```python
from build123d import *

# Parameters (mm, degrees)
F1_DEPTH = 101.6
F3_R     = 1.984375
F4_DEPTH = 25.4
F6_R     = 1.984375
F7_DEPTH = 31.75
F8_DEPTH = 25.4
F9_DEPTH = 12.7


with BuildPart() as f1:
    # F0 (on Front) → F1 (new body)
    with BuildSketch(Plane.XZ):
        with BuildLine():
            Line((114.3, 0), (127, 0))
            ThreePointArc((127, 0), (0, 127), (-127, 0))
            Line((-127, 0), (-114.3, 0))
            ThreePointArc((-114.3, 0), (0, 114.3), (114.3, 0))
        make_face()
    extrude(amount=F1_DEPTH)

    # F3 (on face) → F4 (cut)
    with BuildSketch(Plane(origin=(0, 0, 0), x_dir=(1, 0, 0), z_dir=(0, 0, -1))):
        with Locations((0, 222.573593)):
            Circle(F3_R)
    extrude(amount=-F4_DEPTH, mode=Mode.SUBTRACT)

    # F6 (on offset) → F7 (cut)
    with BuildSketch(Plane.YZ.offset(152.4)):
        with Locations((-12.7, 6.35)):
            Circle(F6_R)
    extrude(amount=-F7_DEPTH, mode=Mode.SUBTRACT)

    # F2 (on face) → F8 (join)
    with BuildSketch(Plane(origin=(0, 0, 0), x_dir=(1, 0, 0), z_dir=(0, 0, -1))):
        with BuildLine():
            ThreePointArc((-114.3, 101.6), (0, 215.9), (114.3, 101.6))
            Line((114.3, 101.6), (127, 101.6))
            ThreePointArc((127, 101.6), (0, 228.6), (-127, 101.6))
            Line((-127, 101.6), (-114.3, 101.6))
        make_face()
    extrude(amount=-F8_DEPTH)

    # F3 (on face) → F9 (cut)
    with BuildSketch(Plane(origin=(0, 0, 0), x_dir=(1, 0, 0), z_dir=(0, 0, -1))):
        with Locations((0, 222.573593)):
            Circle(F3_R)
    extrude(amount=-F9_DEPTH, mode=Mode.SUBTRACT)


solid = f1.part
```
Part model, mm, in its own coordinate system. A direction names the side the tool comes from. Round coordinates to 2 decimals unless told otherwise and drop trailing zeros. Loops run counter-clockwise (first coordinate to the right, second up) from the corner with the lowest first, then second, coordinate; pieces in that order, holes last. Notation, with made-up numbers: (76, -26) -> (112, -26) arc R19 cw to (112, -17) -> close; hole circle Ø11 at (-24, 53.5). An arc over 180 degrees is marked (long way). Use one line per item in the form item = value. Start each with the question number.
Item 1: Drop flat-ended pins along their axis: pin 1 Ø1.5 at (y, z) = (-92.5, 105) entering from +X; pin 2 Ø4 at (x, z) = (-75.5, 91) entering from -Y; pin 3 Ø2 at (x, y) = (0, -223) entering from -Z. Give the stop position or say it passes through.
Item 2: Band-saw the part on C-C (y = -75). List the corners of the cut face in (x, z), plus the area to 3 significant figures.
Item 3: Drill centre lines: line 1 along Y through (x, z) = (0, 3.75); line 2 along Y through (x, z) = (-84, 84.5); line 3 along X through (y, z) = (-71, 28). Where is each one in solid material? Low to high.
Item 4: Band-saw the part on B-B (y = -160.5). List the corners of the cut face in (x, z), plus the area to 3 significant figures.
Item 5: Tool access for faces 4 (the flat face through (-1, -217, 25.4)), 5 (the cylindrical face through (2.79, -228.57, 12.52)), 6 (the cylindrical face through (-2.513, -50.089, 114.272)): list every direction of +Z, -Z, +X, -X, +Y, -Y with a clear straight run to the whole face (end or side of a thin tool).
Item 6: Band-saw the part on D-D (z = 21). List the corners of the cut face in (x, y), plus the area to 3 significant figures.
Item 7: Band-saw the part on A-A (z = 95.5). List the corners of the cut face in (x, y), plus the area to 3 significant figures.
Item 8: Two-plate mould, pull along X, no slides. Class faces 1 (the cylindrical face through (2.79, -50.09, 126.97)), 2 (the flat face through (-1, 0, 116)), 3 (the cylindrical face through (-2.513, -215.872, 12.522)): released by +X, released by -X, zero draft, split by the parting line, or undercut.
Data:
q1.pin_1 = 72.53
q1.pin_2 = -101.6
q1.pin_3 = 12.7
q2.outline = (-127, 0) -> (-114.3, 0) arc R114.3 cw to (114.3, 0) -> (127, 0) arc R127 ccw to start
q2.area = 4,810 mm^2
q3.line_1 = -228.6 to -224.56, -220.59 to -215.9
q3.line_2 = -101.6 to 0
q3.line_3 = -123.87 to -110.82, 110.82 to 123.87
q4.outline = (-112.52, 0) -> (-97.96, 0) -> (-97.96, 25.4) -> (-112.52, 25.4) -> close; (97.96, 0) -> (112.52, 0) -> (112.52, 25.4) -> (97.96, 25.4) -> close
q4.area = 740 mm^2
q5.face_4 = +Z, +X, -X, -Y
q5.face_5 = +Z, -Z, -Y
q5.face_6 = -Z, +Y
q6.outline = (-127, -101.6) arc R127 ccw to (127, -101.6) -> (125.25, -101.6) -> (125.25, 0) -> (112.35, 0) -> (112.35, -101.6) -> (114.3, -101.6) arc R114.3 cw to (-114.3, -101.6) -> (-112.35, -101.6) -> (-112.35, 0) -> (-125.25, 0) -> (-125.25, -101.6) -> close
q6.area = 7,430 mm^2
q7.outline = (-83.72, -101.6) -> (-62.8, -101.6) -> (-62.8, 0) -> (-83.72, 0) -> close; (62.8, -101.6) -> (83.72, -101.6) -> (83.72, 0) -> (62.8, 0) -> close
q7.area = 4,250 mm^2
q8.face_1 = split by the parting line
q8.face_2 = zero draft
q8.face_3 = undercut
